Part model, mm, in its own coordinate system. A direction names the side the tool comes from. Round coordinates to 2 decimals unless told otherwise and drop trailing zeros. Loops run counter-clockwise (first coordinate to the right, second up) from the corner with the lowest first, then second, coordinate; pieces in that order, holes last.
from build123d import *

# Parameters (mm, degrees)
SKETCH1_R           = 1
BOSS_EXTRUDE1_DEPTH = 12
BOSS_EXTRUDE2_START = -2
SKETCH1_3_R         = 2
SKETCH1_3_R_2       = 1
BOSS_EXTRUDE2_DEPTH = 2
CUT_EXTRUDE1_DEPTH  = 2
FILLET1_R           = 0.25


with BuildPart() as part:
    # Sketch1 → Boss-Extrude1 (new body)
    with BuildSketch(Plane(origin=(0, 0, 0), x_dir=(1, 0, 0), z_dir=(0, 1, 0))):
        with Locations(Location((0, 0, 0), (0, 0, 270))):
            Circle(SKETCH1_R)
    extrude(amount=BOSS_EXTRUDE1_DEPTH)

    # Sketch1_3 → Boss-Extrude2 (add)
    # profile 1 of 2: a face of its own
    with BuildSketch(Plane(origin=(0, 0, 0), x_dir=(1, 0, 0), z_dir=(0, 1, 0)).offset(BOSS_EXTRUDE2_START)):
        with Locations(Location((0, 0, 0), (0, 0, 270))):
            Circle(SKETCH1_3_R)
        with Locations(Location((0, 0, 0), (0, 0, 270))):
            Circle(SKETCH1_3_R_2, mode=Mode.SUBTRACT)
    # profile 2 of 2: a face of its own
    with BuildSketch(Plane(origin=(0, 0, 0), x_dir=(1, 0, 0), z_dir=(0, 1, 0)).offset(BOSS_EXTRUDE2_START)):
        with Locations(Location((0, 0, 0), (0, 0, 270))):
            Circle(SKETCH1_3_R_2)
    extrude(amount=BOSS_EXTRUDE2_DEPTH)

    # Sketch2 → Cut-Extrude1 (cut)
    with BuildSketch(Plane.XZ.offset(2)):
        Polygon((0, 0.866025404), (-0.75, 0.433012702), (-0.75, -0.433012702), (0, -0.866025404), (0.75, -0.433012702), (0.75, 0.433012702), align=None)
    extrude(amount=-CUT_EXTRUDE1_DEPTH, mode=Mode.SUBTRACT)

    # Fillet1
    fillet1_edges = [part.edges().sort_by_distance(p)[0] for p in [
        (0, -2, -2),
        (0, 0, -2),
    ]]
    fillet(fillet1_edges, radius=FILLET1_R)


solid = part.part
1) Drop flat-ended pins along their axis: pin 1 Ø1 at (x, y) = (0, 6) entering from +Z; pin 2 Ø1 at (y, z) = (4.5, -1) entering from -X; pin 3 Ø1.7 at (x, z) = (0, 0.5) entering from -Y; pin 4 Ø1 at (y, z) = (8.5, -0.5) entering from +X. Give the stop position or say it passes through.
Values:
pin 1: stops at z = 1
pin 2: stops at x = -0.87
pin 3: stops at y = -2
pin 4: stops at x = 1
2) Slice it at A-A, the plane z = 0. Give the cut face in (x, y).
Values:
outline: (-2, -1.75) arc R0.25 ccw to (-1.75, -2) - (-0.75, -2) - (-0.75, 0) - (0.75, 0) - (0.75, -2) - (1.75, -2) arc R0.25 ccw to (2, -1.75) - (2, -0.25) arc R0.25 ccw to (1.75, 0) - (1, 0) - (1, 12) - (-1, 12) - (-1, 0) - (-1.75, 0) arc R0.25 ccw to (-2, -0.25) - close
3) Tool access for faces 1 (the face through (-1, -2, 0)), 2 (the face through (-1, 6, 0)), 3 (the face through (-0.75, -1, 0)): list every direction of +Z, -Z, +X, -X, +Y, -Y with a clear straight run to the whole face (end or side of a thin tool).
Values:
face 1: +Z, -Z, +X, -X, -Y
face 2: +Y
face 3: -Y
4) Wall check: line 1 along Y through (x, z) = (1.25, 0.35); line 2 along X through (y, z) = (10.75, 0.35); line 3 along X through (y, z) = (5, -0.8). Give the ranges that are in metal, low to high.
Values:
line 1: y = -2 to 0
line 2: x = -0.94 to 0.94
line 3: x = -0.6 to 0.6
5) Slice it at B-B, the plane y = 3.5. Give the cut face in (x, z), then the cut area to 3 significant figures.
Values:
outline: circle Ø2 at (0, 0)
area: 3.14 mm2
